```python
from build123d import *

# Parameters (mm, degrees)
EXTRUDE_1_DEPTH          = 12
CHAMFER_1_SIZE           = 3
SKETCH_2_R               = 4
EXTRUDE_2_DEPTH          = 12
HOLE_WIZARD_1_D          = 4.917
HOLE_WIZARD_1_DEPTH      = 17.1
HOLE_WIZARD_1_TIP        = 1.477215832
SKETCH_5_R               = 4.5
EXTRUDE_4_DEPTH          = 12
SKETCH_6_R               = 4.5
EXTRUDE_3_DEPTH          = 12
SKETCH_7_R               = 4.5
EXTRUDE_5_DEPTH          = 12
MIRROR_2_COPY_1_SKETCH_R = 4.5
MIRROR_2_COPY_1_DEPTH    = 12
SKETCH_8_R               = 4.5
EXTRUDE_8_DEPTH          = 12
SKETCH_9_R               = 4.5
EXTRUDE_9_DEPTH          = 12
MIRROR_8_COPY_1_SKETCH_R = 4.5
MIRROR_8_COPY_1_DEPTH    = 12


with BuildPart() as part:
    # 草圖1 → 擠出1 (new body)
    with BuildSketch(Plane(origin=(0, 0, 0), x_dir=(-1, 0, 0), z_dir=(0, 1, 0))):
        Polygon((0, -86.602540378), (-75, -43.301270189), (-75, 43.301270189), (0, 86.602540378), (75, 43.301270189), (75, -43.301270189), align=None)
    extrude(amount=EXTRUDE_1_DEPTH)

    # 倒角1
    chamfer_1_edges = [part.edges().sort_by_distance(p)[0] for p in [
        (37.5, 0, -64.951905284),
        (75, 0, 0),
        (37.5, 0, 64.951905284),
        (-37.5, 0, 64.951905284),
        (-75, 0, 0),
        (-37.5, 0, -64.951905284),
    ]]
    chamfer(chamfer_1_edges, length=CHAMFER_1_SIZE)

    # 草圖2 → 擠出2 (cut)
    with BuildSketch(Plane(origin=(0, 12, 0), x_dir=(-1, 0, 0), z_dir=(0, 1, 0))):
        with Locations(Location((-32.5, 56.5, 0), (0, 0, 90))):
            Circle(SKETCH_2_R)
        with Locations(Location((32.5, 56.5, 0), (0, 0, 90))):
            Circle(SKETCH_2_R)
        with Locations(Location((-65, 0, 0), (0, 0, 90))):
            Circle(SKETCH_2_R)
        with Locations(Location((-32.5, -56.5, 0), (0, 0, 90))):
            Circle(SKETCH_2_R)
        with Locations(Location((32.5, -56.5, 0), (0, 0, 90))):
            Circle(SKETCH_2_R)
        with Locations(Location((65, 0, 0), (0, 0, 90))):
            Circle(SKETCH_2_R)
    extrude(amount=-EXTRUDE_2_DEPTH, mode=Mode.SUBTRACT)

    # 孔1
    with Locations(Plane(origin=(0, 12, 0), x_dir=(1, 0, 0), z_dir=(0, 1, 0))):
        with Locations((0, 75.5), (-65, 37.5), (65, 37.5), (-65, -37.5), (65, -37.5), (0, -75.5)):
            Hole(HOLE_WIZARD_1_D / 2, depth=HOLE_WIZARD_1_DEPTH)
            with Locations((0, 0, -(HOLE_WIZARD_1_DEPTH + HOLE_WIZARD_1_TIP / 2))):  # 118° drill point
                Cone(0, HOLE_WIZARD_1_D / 2, HOLE_WIZARD_1_TIP, mode=Mode.SUBTRACT)

    # 草圖5 → 擠出4 (cut)
    with BuildSketch(Plane(origin=(0, 12, 0), x_dir=(-1, 0, 0), z_dir=(0, 1, 0))):
        with Locations(Location((0, 0, 0), (0, 0, 90))):
            Circle(SKETCH_5_R)
    extrude(amount=-EXTRUDE_4_DEPTH, mode=Mode.SUBTRACT)

    # 草圖6 → 擠出3 (cut)
    with BuildSketch(Plane(origin=(0, 12, 0), x_dir=(1, 0, 0), z_dir=(0, 1, 0))):
        with Locations(Location((20, 0, 0), (0, 0, 270))):
            Circle(SKETCH_6_R)
        with Locations(Location((35, 0, 0), (0, 0, 270))):
            Circle(SKETCH_6_R)
        with Locations(Location((50, 0, 0), (0, 0, 270))):
            Circle(SKETCH_6_R)
    extrude_3 = extrude(amount=-EXTRUDE_3_DEPTH, mode=Mode.SUBTRACT)

    # 鏡射5: 擠出3 across plane
    add(extrude_3.mirror(Plane(origin=(0, 0, 0), x_dir=(0, 0, 1), z_dir=(1, 0, 0))), mode=Mode.SUBTRACT)

    # 草圖7 → 擠出5 (cut)
    with BuildSketch(Plane(origin=(0, 12, 0), x_dir=(1, 0, 0), z_dir=(0, 1, 0))):
        with Locations(Location((20, 11.5, 0), (0, 0, 270))):
            Circle(SKETCH_7_R)
        with Locations(Location((35, 20, 0), (0, 0, 270))):
            Circle(SKETCH_7_R)
        with Locations(Location((50, 29, 0), (0, 0, 270))):
            Circle(SKETCH_7_R)
    extrude_5 = extrude(amount=-EXTRUDE_5_DEPTH, mode=Mode.SUBTRACT)

    # 鏡射1: 擠出5 across plane
    add(extrude_5.mirror(Plane.XY), mode=Mode.SUBTRACT)

    # 鏡射2: 擠出5 across plane
    add(extrude_5.mirror(Plane(origin=(0, 0, 0), x_dir=(0, 0, 1), z_dir=(1, 0, 0))), mode=Mode.SUBTRACT)

    # 鏡射2 copy 1 sketch → 鏡射2 copy 1 (cut)
    with BuildSketch(Plane(origin=(0, 12, 0), x_dir=(-1, 0, 0), z_dir=(0, 1, 0))):
        with Locations(Location((20, 11.5, 0), (0, 0, 270))):
            Circle(MIRROR_2_COPY_1_SKETCH_R)
        with Locations(Location((35, 20, 0), (0, 0, 270))):
            Circle(MIRROR_2_COPY_1_SKETCH_R)
        with Locations(Location((50, 29, 0), (0, 0, 270))):
            Circle(MIRROR_2_COPY_1_SKETCH_R)
    extrude(amount=-MIRROR_2_COPY_1_DEPTH, mode=Mode.SUBTRACT)

    # 草圖8 → 擠出8 (cut)
    with BuildSketch(Plane(origin=(0, 12, 0), x_dir=(1, 0, 0), z_dir=(0, 1, 0))):
        with Locations(Location((0, -23.047005384, 0), (0, 0, 270))):
            Circle(SKETCH_8_R)
        with Locations(Location((0, -40.207259422, 0), (0, 0, 270))):
            Circle(SKETCH_8_R)
        with Locations(Location((0, -57.867513459, 0), (0, 0, 270))):
            Circle(SKETCH_8_R)
    extrude_8 = extrude(amount=-EXTRUDE_8_DEPTH, mode=Mode.SUBTRACT)

    # 鏡射6: 擠出8 across plane
    add(extrude_8.mirror(Plane.XY), mode=Mode.SUBTRACT)

    # 草圖9 → 擠出9 (cut)
    with BuildSketch(Plane(origin=(0, 12, 0), x_dir=(1, 0, 0), z_dir=(0, 1, 0))):
        with Locations(Location((10, -17.273502692, 0), (0, 0, 270))):
            Circle(SKETCH_9_R)
        with Locations(Location((17.5, -30.353629711, 0), (0, 0, 270))):
            Circle(SKETCH_9_R)
        with Locations(Location((25, -43.43375673, 0), (0, 0, 270))):
            Circle(SKETCH_9_R)
    extrude_9 = extrude(amount=-EXTRUDE_9_DEPTH, mode=Mode.SUBTRACT)

    # 鏡射7: 擠出9 across plane
    add(extrude_9.mirror(Plane(origin=(0, 0, 0), x_dir=(0, 0, 1), z_dir=(1, 0, 0))), mode=Mode.SUBTRACT)

    # 鏡射8: 擠出9 across plane
    add(extrude_9.mirror(Plane.XY), mode=Mode.SUBTRACT)

    # 鏡射8 copy 1 sketch → 鏡射8 copy 1 (cut)
    with BuildSketch(Plane(origin=(0, 12, 0), x_dir=(-1, 0, 0), z_dir=(0, 1, 0))):
        with Locations(Location((10, -17.273502692, 0), (0, 0, 270))):
            Circle(MIRROR_8_COPY_1_SKETCH_R)
        with Locations(Location((17.5, -30.353629711, 0), (0, 0, 270))):
            Circle(MIRROR_8_COPY_1_SKETCH_R)
        with Locations(Location((25, -43.43375673, 0), (0, 0, 270))):
            Circle(MIRROR_8_COPY_1_SKETCH_R)
    extrude(amount=-MIRROR_8_COPY_1_DEPTH, mode=Mode.SUBTRACT)


solid = part.part
```
Check sheet for the modelled part. Datum: model origin and axes. Units: mm. Coordinates: 2 decimals unless noted, no trailing zeros. Write each loop counter-clockwise with the first axis right and the second up, starting at its lowest first coordinate (ties: lowest second). Pieces come first, ordered by that corner, then holes. Notation, with made-up numbers: M 42.5,44 L 75.5,44 A12 ccw 75.5,53 Z; hole C -23.5,-37.5 d2. An arc over 180 degrees is marked long. Use one line per item in the form item = value.
Item 1: Sectioned sample at D-D, the plane x = 32.5. Record the cut outline in (y, z), and give its area (3 significant figures).
Answer below:
outline = M 0,-64.37 L 3,-67.84 L 12,-67.84 L 12,-60.5 L 0,-60.5 Z; M 0,-52.5 L 12,-52.5 L 12,-23.74 L 0,-23.74 Z; M 0,-16.26 L 12,-16.26 L 12,-3.74 L 0,-3.74 Z; M 0,3.74 L 12,3.74 L 12,16.26 L 0,16.26 Z; M 0,23.74 L 12,23.74 L 12,52.5 L 0,52.5 Z; M 0,60.5 L 12,60.5 L 12,67.84 L 3,67.84 L 0,64.37 Z
area = 1,160 mm^2
Item 2: Sectioned sample at B-B, the plane z = 0. State how many separate pieces and enclosed holes the cut face has, and give its area (3 significant figures).
Answer below:
separate_pieces = 10
enclosed_holes = 0
area = 843 mm^2
Item 3: Sectioned sample at C-C, the plane x = -10. Record the cut outline in (y, z), and give its area (3 significant figures).
Answer below:
outline = M 0,-77.36 L 3,-80.83 L 12,-80.83 L 12,-21.77 L 0,-21.77 Z; M 0,-12.77 L 12,-12.77 L 12,12.77 L 0,12.77 Z; M 0,21.77 L 12,21.77 L 12,80.83 L 3,80.83 L 0,77.36 Z
area = 1,710 mm^2
Item 4: Sectioned sample at A-A, the plane x = -50. Record the cut outline in (y, z).
Answer below:
outline = M 0,-54.27 L 3,-57.74 L 12,-57.74 L 12,-33.5 L 0,-33.5 Z; M 0,-24.5 L 12,-24.5 L 12,-4.5 L 0,-4.5 Z; M 0,4.5 L 12,4.5 L 12,24.5 L 0,24.5 Z; M 0,33.5 L 12,33.5 L 12,57.74 L 3,57.74 L 0,54.27 Z
Item 5: Release check for a two-part mould opening along X. For faces 1 (the face through (36.975, 7.437, -65.255)), 2 (the face through (-29.127, 6.084, 58.65)), 3 (the face through (-38.02, 7.44, -64.65)) record: pulls with the +X half, pulls with the -X half, needs draft (parallel to the pull), parting line crosses it, or undercut.
Answer below:
face_1 = pulls with the +X half
face_2 = undercut
face_3 = pulls with the -X half
Item 6: Gauge pin test, flat ends, axial feed: pin 1 Ø6 at (x, y) = (28.5, 5.5) entering from -Z; pin 2 Ø1 at (y, z) = (1.5, -29.5) entering from +X; pin 3 Ø5.5 at (x, z) = (0, -75.5) entering from -Y; pin 4 Ø1.5 at (x, y) = (14, 5) entering from +Z. Record the tip position at first contact, or that the pin passes through.
Answer below:
pin_1 = -71.88
pin_2 = 74
pin_3 = 0
pin_4 = 78.95
Item 7: Material ranges on L1, parallel to Z at x = -50, y = 4; L2, parallel to Z at x = -17.5, y = 6.75; L3, parallel to Z at x = 51, y = 5.25, recorded low to high. Write a range as from..to.
Answer below:
L1 = -57.74..-33.5, -24.5..-4.5, 4.5..24.5, 33.5..57.74
L2 = -76.5..-34.85, -25.85..-15.24, -7.76..-3.74, 3.74..7.76, 15.24..25.85, 34.85..76.5
L3 = -57.16..-33.39, -24.61..-4.39, 4.39..24.61, 33.39..57.16
